Answer from the drawing. Dimensions are ordinates in mm from the lowest x, y and z of the part. A direction names the side the tool comes from. Coordinates: 2 decimals unless noted, no trailing zeros. Order: outer loops, then holes, each group sorted by start corner. A loop starts at its lowest first (then second) coordinate and runs counter-clockwise, first axis right, second up. Notation, with made-up numbers: (61.25, 16) -> (97.25, 16) arc R10 ccw to (97.25, 32) -> close; hole circle Ø4 at (15.5, 19.5). An arc over 180 degrees is marked (long way). Answer as a JSON object with one key per item and string values. Group by question number.
1) Section B-B on z = 102.5 is taken. Determine the outline of the cut face in (x, y).
2) Section C-C on y = 67.5 is taken. Determine the outline of the cut face in (x, z).
3) Section A-A on x = 70 is taken. Determine the outline of the cut face in (y, z).
4) A tool of negligible diameter and unlimited length cuts with its end or side. For the marked faces 1 and 2, from which of +Z, -Z, +X, -X, +Y, -Y can it reach the whole face along a straight path? Write none if from no direction.
5) Given pin 1 (3 mm diameter, centred on y = 76, z = 45, fed in from -X); pin 2 (12 mm diameter, centred on x = 76, y = 62.5, fed in from -Z); pin 3 (10 mm diameter, centred on y = 95, z = 37.5, fed in from +X), each flat-ended and moving along its own axis, determine where each tip first touches the part or whether it passes through.
6) Consider L1, parallel to Y at x = 73, z = 61; L2, parallel to X at y = 55, z = 50; L3, parallel to Z at x = 76, y = 22.5. Determine where each line is inside the solid, lowest interval first.
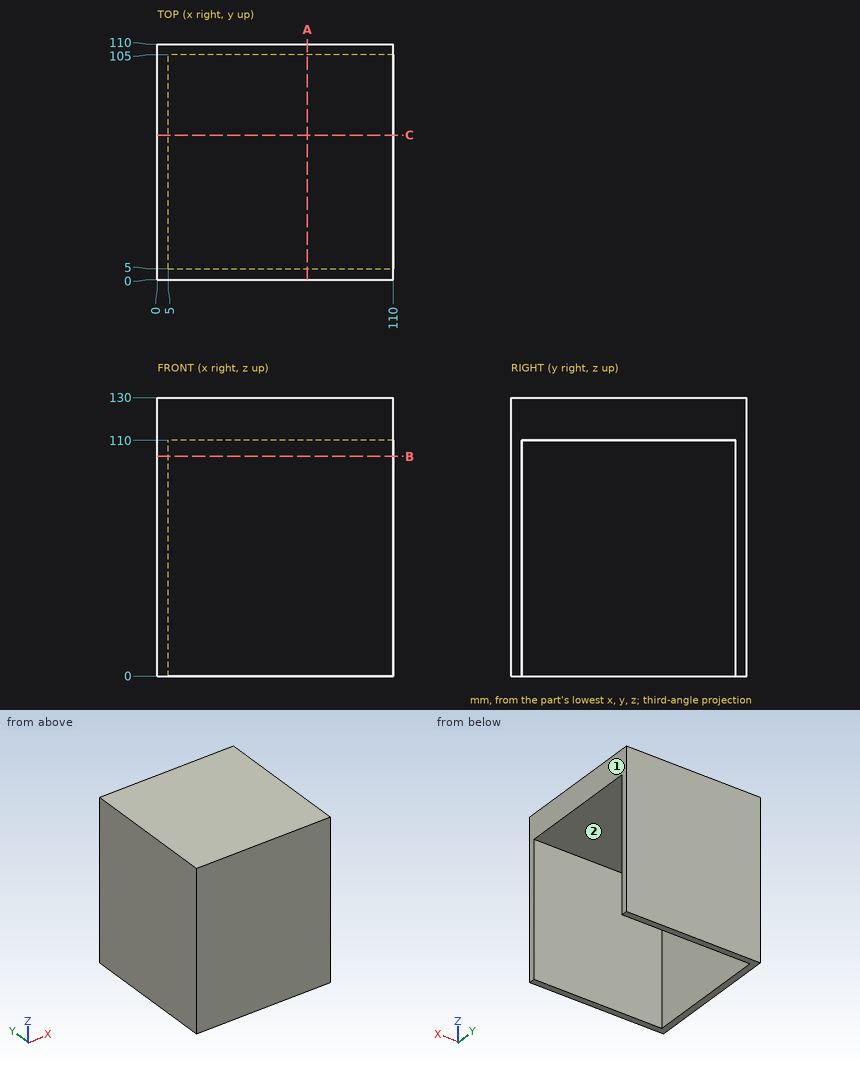
Worked answers:
{
 "1": {"outline": "(0, 0) -> (110, 0) -> (110, 5) -> (5, 5) -> (5, 105) -> (110, 105) -> (110, 110) -> (0, 110) -> close"},
 "2": {"outline": "(0, 0) -> (5, 0) -> (5, 110) -> (110, 110) -> (110, 130) -> (0, 130) -> close"},
 "3": {"outline": "(0, 0) -> (5, 0) -> (5, 110) -> (105, 110) -> (105, 0) -> (110, 0) -> (110, 130) -> (0, 130) -> close"},
 "4": {"face 1": "+Z, -Z, +X, +Y, -Y", "face 2": "-Z, +X"},
 "5": {"pin 1": "stops at x = 0", "pin 2": "stops at z = 110", "pin 3": "stops at x = 5"},
 "6": {"L1": "y = 0 to 5, 105 to 110", "L2": "x = 0 to 5", "L3": "z = 110 to 130"}
}
